Source: CAD feature listing. Evaluate the final solid. Frame: model axes, mm. Face numbers are marked on the shaded views. A direction names the side the tool comes from. Coordinates: 2 decimals unless noted, no trailing zeros. Write each loop counter-clockwise with the first axis right and the second up, starting at its lowest first coordinate (ties: lowest second). Pieces come first, ordered by that corner, then holes. Notation, with made-up numbers: (-28, 52) - (-10, 52) arc R7 ccw to (-10, 57) - close; hole circle Ø4 at (-19.75, 65.25). An arc over 180 degrees is marked (long way). One line per item, written item: value.
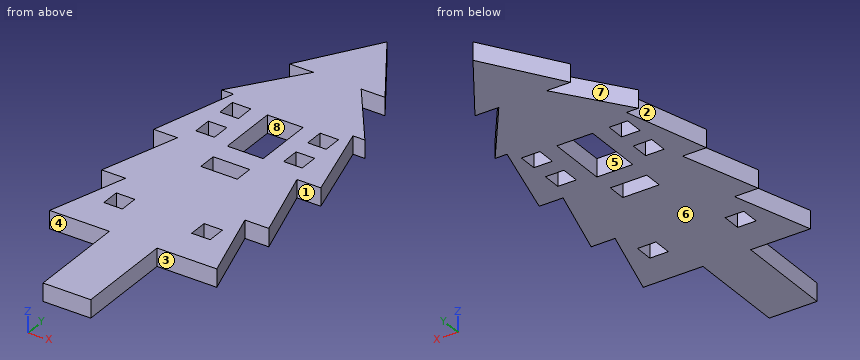
from build123d import *

# Parameters (mm, degrees)
PROFILE_LASER_PROFILE_3MM_W   = 3.1
PROFILE_LASER_PROFILE_3MM_H   = 3.1
PROFILE_LASER_PROFILE_3MM_W_2 = 6.1
PROFILE_LASER_PROFILE_3MM_W_3 = 6
PROFILE_LASER_PROFILE_3MM_H_2 = 10
LASER_PROFILE_3MM_DEPTH       = 3


with BuildPart() as part:
    # Profile_Laser_profile_3mm → Laser_profile_3mm (new body)
    with BuildSketch(Plane.XY):
        Polygon((0, 30.427227289), (8, 18), (4, 18), (12, 7), (10, 7), (14, -7), (10, -7), (14, -20), (10, -20), (14, -33), (4, -33), (4, -49.572772711), (-4, -49.572772711), (-4, -33), (-14, -33), (-10, -20), (-14, -20), (-10, -7), (-14, -7), (-10, 7), (-12, 7), (-4, 18), (-8, 18), align=None)
        with Locations((-7.35, 3.5)):
            Rectangle(PROFILE_LASER_PROFILE_3MM_W, PROFILE_LASER_PROFILE_3MM_H, mode=Mode.SUBTRACT)
        with Locations((-7.35, -2.5)):
            Rectangle(PROFILE_LASER_PROFILE_3MM_W, PROFILE_LASER_PROFILE_3MM_H, mode=Mode.SUBTRACT)
        with Locations((-7.35, -25.5)):
            Rectangle(PROFILE_LASER_PROFILE_3MM_W, PROFILE_LASER_PROFILE_3MM_H, mode=Mode.SUBTRACT)
        with Locations((7.35, 3.5)):
            Rectangle(PROFILE_LASER_PROFILE_3MM_W, PROFILE_LASER_PROFILE_3MM_H, mode=Mode.SUBTRACT)
        with Locations((7.35, -2.5)):
            Rectangle(PROFILE_LASER_PROFILE_3MM_W, PROFILE_LASER_PROFILE_3MM_H, mode=Mode.SUBTRACT)
        with Locations((7.35, -25.5)):
            Rectangle(PROFILE_LASER_PROFILE_3MM_W, PROFILE_LASER_PROFILE_3MM_H, mode=Mode.SUBTRACT)
        with Locations((0, -10)):
            Rectangle(PROFILE_LASER_PROFILE_3MM_W_2, PROFILE_LASER_PROFILE_3MM_H, mode=Mode.SUBTRACT)
        Rectangle(PROFILE_LASER_PROFILE_3MM_W_3, PROFILE_LASER_PROFILE_3MM_H_2, mode=Mode.SUBTRACT)
    extrude(amount=LASER_PROFILE_3MM_DEPTH)


solid = part.part
1) Section query D-D on y = -41.5. Output: boundary loops of the cut face in (x, z), then the cut area to 3 significant figures.
Values found:
outline: (-4, 0) - (4, 0) - (4, 3) - (-4, 3) - close
area: 24.0 mm2
2) Section query B-B on z = 2.55. State how many separate pieces and enclosed holes the cut face has, then the cut area to 3 significant figures.
Values found:
separate pieces: 1
enclosed holes: 8
area: 1,230 mm2
3) Section query A-A on x = 2. Output: boundary loops of the cut face in (y, z).
Values found:
outline: (-49.57, 0) - (-11.55, 0) - (-11.55, 3) - (-49.57, 3) - close; (-8.45, 0) - (-5, 0) - (-5, 3) - (-8.45, 3) - close; (5, 0) - (27.32, 0) - (27.32, 3) - (5, 3) - close
4) Draft query along X for the marked faces 5, 6, 7 and 8. Return one class per face: released by +X, released by -X, zero draft, split by the parting line, or undercut.
Values found:
face 5: undercut
face 6: zero draft
face 7: released by -X
face 8: undercut
5) Reachability of the marked faces 1, 2, 3 and 4 from +Z, -Z, +X, -X, +Y, -Y: full face, straight path, thin tool, end or side. Return the list, or none.
Values found:
face 1: +Z, -Z, +X
face 2: +Z, -Z, -X
face 3: +Z, -Z, +X, -Y
face 4: +Z, -Z, -X, -Y
6) Contact query for flat-ended pins moving along their axis: P1, Ø1.5, axis at x = -6.5, z = 1, coming from the +Y side; P2, Ø1.5, axis at y = -26, z = 1.5, coming from the -X side; P3, Ø1, axis at x = 7.5, z = 1.5, coming from the -Y side. Output: stop coordinate, or through.
Values found:
P1: y = 21.5
P2: x = -12.08
P3: y = -33
7) Section query C-C on x = 11.25. Output: boundary loops of the cut face in (y, z) (1 decimal), then the cut area to 3 significant figures.
Values found:
outline: (-33, 0) - (-24.1, 0) - (-24.1, 3) - (-33, 3) - close; (-20, 0) - (-11.1, 0) - (-11.1, 3) - (-20, 3) - close; (-7, 0) - (2.6, 0) - (2.6, 3) - (-7, 3) - close; (7, 0) - (8, 0) - (8, 3) - (7, 3) - close
area: 85.6 mm2
8) Material intervals for line 1 (Y direction, x = -7.25, z = 0.4); line 2 (Y direction, x = 0.25, z = 1.4); line 3 (Y direction, x = -1.5, z = 2.25), sorted ascending.
Values found:
line 1: -33 to -27.05, -23.95 to -4.05, -0.95 to 1.95, 5.05 to 13.53, 18 to 19.17
line 2: -49.57 to -11.55, -8.45 to -5, 5 to 30.04
line 3: -49.57 to -11.55, -8.45 to -5, 5 to 28.1
